from build123d import *

# Parameters (mm, degrees)
SKETCH1_R               = 41.25
SKETCH1_R_2             = 37.75
BOSS_EXTRUDE1_DEPTH     = 15
SKETCH2_R               = 2
CUT_EXTRUDE2_DEPTH      = 50
CUT_EXTRUDE2_DEPTH_BACK = 50
SKETCH4_R               = 2
CUT_EXTRUDE3_DEPTH      = 50
CUT_EXTRUDE3_DEPTH_BACK = 50


with BuildPart() as part:
    # Sketch1 → Boss-Extrude1 (new body)
    with BuildSketch(Plane(origin=(0, 0, 0), x_dir=(1, 0, 0), z_dir=(0, 1, 0))):
        Circle(SKETCH1_R)
        Circle(SKETCH1_R_2, mode=Mode.SUBTRACT)
    extrude(amount=BOSS_EXTRUDE1_DEPTH)

    # Sketch2 → Cut-Extrude2 (cut, two sides)
    with BuildSketch(Plane(origin=(0, 0, 0), x_dir=(0, 0, -1), z_dir=(1, 0, 0))) as cut_extrude2_sk:
        with Locations((0, 7.5)):
            Circle(SKETCH2_R)
    extrude(amount=CUT_EXTRUDE2_DEPTH, mode=Mode.SUBTRACT)
    extrude(cut_extrude2_sk.sketch, amount=-CUT_EXTRUDE2_DEPTH_BACK, mode=Mode.SUBTRACT)

    # Sketch4 → Cut-Extrude3 (cut, two sides)
    with BuildSketch(Plane.XY) as cut_extrude3_sk:
        with Locations((0, 7.5)):
            Circle(SKETCH4_R)
    extrude(amount=CUT_EXTRUDE3_DEPTH, mode=Mode.SUBTRACT)
    extrude(cut_extrude3_sk.sketch, amount=-CUT_EXTRUDE3_DEPTH_BACK, mode=Mode.SUBTRACT)


solid = part.part
Geometry: final body of the model. Coordinates: model frame, mm. Coordinates: 2 decimals unless noted, no trailing zeros. Loops run counter-clockwise (first coordinate to the right, second up) from the corner with the lowest first, then second, coordinate; pieces in that order, holes last. Notation, with made-up numbers: (65, 35.5) - (92, 35.5) arc R22 cw to (92, 64.5) - close; hole circle Ø7 at (-26, 35.25). An arc over 180 degrees is marked (long way). Put each result on its own line as item: value. Start each with the question number.
Q1. Line query: line 1 (X direction, y = 5, z = 0); line 2 (Y direction, x = -39.8, z = 0). Output: solid intervals per line, ascending.
Q2. Cut plane C-C, the plane x = 13. Return loops of the section in (y, z), and give its area (3 significant figures).
Q3. Cut plane B-B, the plane z = 0. Return loops of the section in (x, y).
Q4. Cut plane D-D, the plane z = 21. Return loops of the section in (x, y).
Q5. Pull-direction query (X, two-part tool) for faces 1 (the cylindrical face through (-39.449, 9.483, 0.26)), 2 (the cylindrical face through (-0.26, 9.483, -39.448)), 3 (the cylindrical face through (36.007, 7.395, -11.339)), 4 (the cylindrical face through (38.105, 7.395, 15.799)); classes: released by +X, released by -X, zero draft, split by the parting line, or undercut.
Q6. Cut plane A-A, the plane x = 0. Return loops of the section in (y, z).
Q7. Pin query (flat end, axial travel): pin 1 Ø4.5 at (x, y) = (0, 7.5) entering from +Z; pin 2 Ø1.5 at (y, z) = (12, 7) entering from -X; pin 3 Ø6 at (y, z) = (11, -32.5) entering from -X; pin 4 Ø5 at (y, z) = (6.5, -3) entering from -X. Return the tip coordinate at first contact, or that it passes through.
Filled sheet:
1. line 1: -41.25 to -37.75, 37.75 to 41.25
1. line 2: 0 to 5.5, 9.5 to 15
2. outline: (0, -39.15) - (15, -39.15) - (15, -35.44) - (0, -35.44) - close; (0, 35.44) - (15, 35.44) - (15, 39.15) - (0, 39.15) - close
2. area: 111 mm²
3. outline: (-41.25, 0) - (-37.75, 0) - (-37.75, 5.5) - (-41.25, 5.5) - close; (-41.25, 9.5) - (-37.75, 9.5) - (-37.75, 15) - (-41.25, 15) - close; (37.75, 0) - (41.25, 0) - (41.25, 5.5) - (37.75, 5.5) - close; (37.75, 9.5) - (41.25, 9.5) - (41.25, 15) - (37.75, 15) - close
4. outline: (-35.5, 0) - (-31.37, 0) - (-31.37, 15) - (-35.5, 15) - close; (31.37, 0) - (35.5, 0) - (35.5, 15) - (31.37, 15) - close
5. face 1: zero draft
5. face 2: undercut
5. face 3: undercut
5. face 4: split by the parting line
6. outline: (0, -41.25) - (5.5, -41.25) - (5.5, -37.75) - (0, -37.75) - close; (0, 37.75) - (5.5, 37.75) - (5.5, 41.25) - (0, 41.25) - close; (9.5, -41.25) - (15, -41.25) - (15, -37.75) - (9.5, -37.75) - close; (9.5, 37.75) - (15, 37.75) - (15, 41.25) - (9.5, 41.25) - close
7. pin 1: z = 41.25
7. pin 2: x = -40.77
7. pin 3: x = -28.83
7. pin 4: x = -41.24
